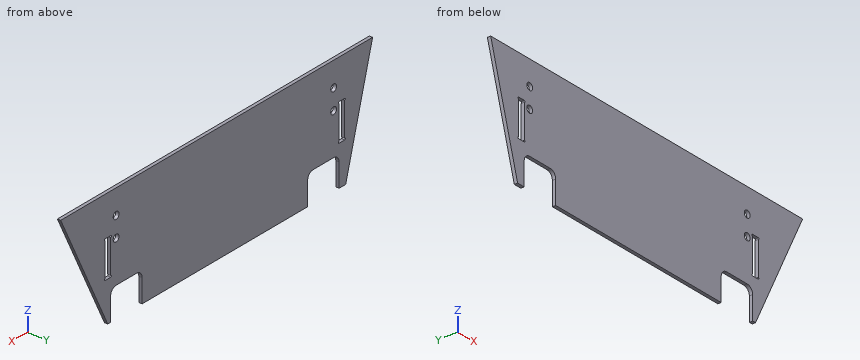
from build123d import *

# Parameters (mm, degrees)
SKETCH1_W               = 361.95
SKETCH1_H               = 110.744
BOSS_EXTRUDE1_DEPTH     = 3.175
CUT_EXTRUDE1_DEPTH      = 4.175
SKETCH3_W               = 36.5125
SKETCH3_H               = 28.575
CUT_EXTRUDE2_DEPTH      = 4.175
FILLET1_R               = 6.35
F_1_4_CLEARANCE_HOLE1_D = 6.7564
SKETCH7_W               = 6.604
SKETCH7_H               = 35.117637185
CUT_EXTRUDE4_DEPTH      = 4.175
SKETCH8_R               = 0.79375
CUT_EXTRUDE5_DEPTH      = 4.175


with BuildPart() as part:
    # Sketch1 → Boss-Extrude1 (new body)
    with BuildSketch(Plane(origin=(0, 0, 0), x_dir=(1, 0, 0), z_dir=(0, 1, 0))):
        with Locations((180.975, 55.372)):
            Rectangle(SKETCH1_W, SKETCH1_H)
    extrude(amount=BOSS_EXTRUDE1_DEPTH)

    # Sketch2 → Cut-Extrude1 (cut, through all)
    with BuildSketch(Plane(origin=(0, 3.175, 0), x_dir=(1, 0, 0), z_dir=(0, 1, 0))):
        Polygon((0, 0), (31.233038214, 110.744), (0, 110.744), align=None)
        Polygon((361.95, 0), (307.33710294, 110.744), (361.95, 110.744), align=None)
    extrude(amount=-CUT_EXTRUDE1_DEPTH, mode=Mode.SUBTRACT)

    # Sketch3 → Cut-Extrude2 (cut, through all)
    with BuildSketch(Plane(origin=(0, 3.175, 0), x_dir=(1, 0, 0), z_dir=(0, 1, 0))):
        with Locations((57.15, 96.4565)):
            Rectangle(SKETCH3_W, SKETCH3_H)
        with Locations((285.75, 96.4565)):
            Rectangle(SKETCH3_W, SKETCH3_H)
    extrude(amount=-CUT_EXTRUDE2_DEPTH, mode=Mode.SUBTRACT)

    # Fillet1
    fillet1_edges = [part.edges().sort_by_distance(p)[0] for p in [
        (75.40625, 1.5875, -82.169),
        (38.89375, 1.5875, -82.169),
        (304.00625, 1.5875, -82.169),
        (267.49375, 1.5875, -82.169),
    ]]
    fillet(fillet1_edges, radius=FILLET1_R)

    # 1/4 Clearance Hole1 (through all)
    with Locations(Plane(origin=(0, 3.175, 0), x_dir=(1, 0, 0), z_dir=(0, 1, 0))):
        with Locations((297.65625, 42.364421689), (297.65625, 23.314421689), (45.24375, 23.314421689), (45.24375, 42.559885057)):
            Hole(F_1_4_CLEARANCE_HOLE1_D / 2)

    # Sketch7 → Cut-Extrude4 (cut, through all)
    with BuildSketch(Plane(origin=(0, 3.175, 0), x_dir=(1, 0, 0), z_dir=(0, 1, 0))):
        with Locations((307.18125, 55.212181407)):
            Rectangle(SKETCH7_W, SKETCH7_H)
        with Locations((35.71875, 55.212181407)):
            Rectangle(SKETCH7_W, SKETCH7_H)
    extrude(amount=-CUT_EXTRUDE4_DEPTH, mode=Mode.SUBTRACT)

    # Sketch8 → Cut-Extrude5 (cut, through all)
    with BuildSketch(Plane(origin=(0, 3.175, 0), x_dir=(1, 0, 0), z_dir=(0, 1, 0))):
        with Locations((39.02075, 38.447112815)):
            Circle(SKETCH8_R)
        with Locations((39.02075, 71.97725)):
            Circle(SKETCH8_R)
        with Locations((32.41675, 71.97725)):
            Circle(SKETCH8_R)
        with Locations((32.41675, 38.447112815)):
            Circle(SKETCH8_R)
        with Locations((303.87925, 71.97725)):
            Circle(SKETCH8_R)
        with Locations((310.48325, 71.97725)):
            Circle(SKETCH8_R)
        with Locations((310.48325, 38.447112815)):
            Circle(SKETCH8_R)
        with Locations((303.87925, 38.447112815)):
            Circle(SKETCH8_R)
    extrude(amount=-CUT_EXTRUDE5_DEPTH, mode=Mode.SUBTRACT)


solid = part.part
The listing builds one solid part. Answer for the finished solid, in the listing's coordinates (mm). Give positions to 0.01 mm unless a question says otherwise; leave off trailing zeros. Write each loop counter-clockwise with the first axis right and the second up, starting at its lowest first coordinate (ties: lowest second). Pieces come first, ordered by that corner, then holes.
Item 1: Section A-A, the plane z = -59.5 is taken. Write down the section's boundary in (x, y) (3 decimals).
Item 2: Section C-C, the plane z = -32.5 is taken. Write down the section's boundary in (x, y) (3 decimals), plus the area to 3 significant figures.
Item 3: Find the intervals of material crossed by line 1 along X through (y, z) = (2, -70); line 2 along X through (y, z) = (1.55, -57); line 3 along X through (y, z) = (0.2, -43), in increasing order.
Item 4: Section B-B, the plane y = 0.5 is taken. Count the separate pieces of the cut face and the enclosed holes in it, plus the area to 3 significant figures.
Item 5: Flat-ended cylindrical pins translate along their axes: P1, Ø1, axis at y = 1.5, z = -50, coming from the +X side; P2, Ø1.6, axis at x = 52.5, y = 1, coming from the -Z side; P3, Ø1.6, axis at y = 2, z = -61.5, coming from the -X side. Find the tip coordinate at first contact, or state that the pin passes through.
Item 6: Section D-D, the plane z = -77 is taken. Write down the section's boundary in (x, y) (3 decimals).
Completed:
1. outline: (16.781, 0) - (32.417, 0) - (32.417, 3.175) - (16.781, 3.175) - close; (39.021, 0) - (303.879, 0) - (303.879, 3.175) - (39.021, 3.175) - close; (310.483, 0) - (332.608, 0) - (332.608, 3.175) - (310.483, 3.175) - close
2. outline: (9.166, 0) - (345.923, 0) - (345.923, 3.175) - (9.166, 3.175) - close
2. area: 1,070 mm2
3. line 1: x = 19.74 to 32.42, 39.02 to 303.88, 310.48 to 327.43
3. line 2: x = 16.08 to 32.42, 39.02 to 303.88, 310.48 to 333.84
3. line 3: x = 12.13 to 32.42, 39.02 to 41.89, 48.59 to 294.34, 300.97 to 303.88, 310.48 to 340.74
4. separate pieces: 1
4. enclosed holes: 6
4. area: 32,700 mm2
5. P1: stops at x = 337.54
5. P2: stops at z = -82.17
5. P3: stops at x = 17.12
6. outline: (21.716, 0) - (323.978, 0) - (323.978, 3.175) - (21.716, 3.175) - close
